For this review, take the finished solid that the model builds, in its own axes (mm). Face numbers are marked on the shaded views. A direction names the side the tool comes from. Give positions to 0.01 mm unless a question says otherwise; leave off trailing zeros. Order: outer loops, then holes, each group sorted by start corner. A loop starts at its lowest first (then second) coordinate and runs counter-clockwise, first axis right, second up.
Item 1: Consider section B-B (y = 2.5). Give the boundary of the cut face in (x, z), plus the area to 3 significant figures.
Item 2: For P1, Ø6, axis at x = 5, y = 3, coming from the +Z side; P2, Ø1.5, axis at y = 3, z = -7.5, coming from the +X side, all flat-tipped, find the tip position at first contact; note any pin that passes through.
Item 3: Consider section A-A (x = 19.05). Give the boundary of the cut face in (y, z), plus the area to 3 significant figures.
Item 4: Consider section C-C (z = -6.5). Give the boundary of the cut face in (x, y), plus the area to 3 significant figures.
Item 5: Consider section D-D (z = -13.5). Give the boundary of the cut face in (x, y) (3 decimals).
Item 6: The part is to be moulded in two halves that separate along Y. For the marked faces 1, 2 and 3, say which applies: released by +Y, released by -Y, zero draft, split by the parting line, or undercut.
Item 7: Machinability: for the marked faces 4 and 5, which of the approach directions +Z, -Z, +X, -X, +Y, -Y give a long, thin tool a straight path to every point of the face, cutting with its end or side? Answer none if there is none.
Item 8: For probe 1 along Z at (x, y) = (3, 10.5); probe 2 along Y at (x, z) = (19.05, -12.55); probe 3 along Z at (x, y) = (12.25, 12.25), list the stretches that pass through material, from the lowest coordinate up.
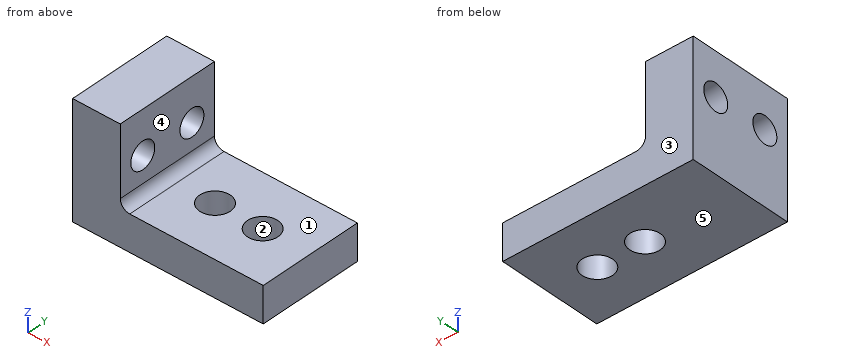
Autodesk Inventor part; units mm, degrees
ref_plane "YZ Plane" through (0, 0, 0) normal (1, 0, 0) x (0, 1, 0)
ref_plane "XZ Plane" through (0, 0, 0) normal (0, 1, 0) x (-1, 0, 0)
ref_plane "XY Plane" through (0, 0, 0) normal (0, 0, 1) x (1, 0, 0)
sketch "Sketch1" plane through (0, 0, 0) normal (1, 0, 0) x (0, 1, 0)
  line L0 (0, 0) -> (13.97, 0)
  line L1 (13.97, 0) -> (13.97, -15.24)
  line L2 (13.97, -15.24) -> (0, -15.24)
  line L3 (0, -15.24) -> (0, 0)
  dimension "d0" = 13.97
  dimension "d1" = 15.24
extrude "Extrusion1" add sketch "Sketch1" along normal blind 6.35
sketch "Sketch2" plane through (6.35, 0, 0) normal (1, 0, 0) x (0, 0, -1)
  line L0 (15.24, 0) -> (15.24, 13.97)
  line L1 (0, 0) -> (15.24, 0)
  line L2 (15.24, 13.97) -> (10.4775, 13.97)
  line L3 (10.4775, 13.97) -> (10.4775, 0)
  line L4 (10.4775, 0) -> (15.24, 0)
  line L5 (15.24, 0) -> (15.24, 13.97)
  dimension "d4" = 4.7625
extrude "Extrusion2" add sketch "Sketch2" along normal blind 19.05
sketch "Sketch3" plane through (6.35, 0, 0) normal (1, 0, 0) x (0, 0, -1)
  line L0 (15.24, 0) -> (0, 0)
  line L1 (0, 0) -> (5.715, 0)
  line L2 (5.715, 0) -> (5.715, 3.3401)
  line L3 (0, 13.97) -> (15.24, 13.97)
  line L4 (5.715, 13.97) -> (5.715, 10.6299)
  line L5 (0, 13.97) -> (0, 0)
  line L6 (15.24, 0) -> (15.24, 13.97)
  dimension "d28" = 9.525
  dimension "d29" = 9.525
  dimension "d30" = 7.2898
  dimension "d31" = 3.3401
  dimension "d32" = 13.97
hole "Hole1" at (6.35, 10.6299, -5.715) at (6.35, 3.3401, -5.715) direction (-1, 0, 0) diameter 3.556 depth 25.4 tip angle 118
fillet "Fillet1" radius 1.27 1 edges at (6.35, 6.985, -10.4775)
sketch "Sketch4" plane through (25.4, 0, -10.4775) normal (0, 0, 1) x (1, 0, 0)
  line L0 (-17.78, 0) -> (0, 0)
  line L1 (0, 0) -> (0, 6.985)
  line L2 (0, 13.97) -> (0, 0)
  line L3 (0, 6.985) -> (-6.35, 6.985)
  line L4 (-19.05, 13.97) -> (-19.05, 0)
  line L5 (-19.05, 6.985) -> (-12.7, 6.985)
  point P0 (-25.4, 0)
  dimension "d19" = 6.35
  dimension "d20" = 6.35
hole "Hole2" at (19.05, 6.985, -10.4775) at (12.7, 6.985, -10.4775) direction (0, 0, -1) diameter 4.064 depth 25.4 tip angle 118
properties part number "GlyphLiftHolder1"
Resolved:
1. outline: (0, -15.24) - (25.4, -15.24) - (25.4, -10.48) - (7.62, -10.48) arc R1.27 cw to (6.35, -9.21) - (6.35, -7.28) - (0, -7.28) - close; (0, -4.15) - (6.35, -4.15) - (6.35, 0) - (0, 0) - close
1. area: 168 mm2
2. P1: stops at z = 0
2. P2: stops at x = 6.35
3. outline: (0, -15.24) - (4.95, -15.24) - (4.95, -10.48) - (0, -10.48) - close; (9.02, -15.24) - (13.97, -15.24) - (13.97, -10.48) - (9.02, -10.48) - close
3. area: 47.2 mm2
4. outline: (0, 0) - (6.35, 0) - (6.35, 1.74) - (0, 1.74) - close; (0, 4.94) - (6.35, 4.94) - (6.35, 9.03) - (0, 9.03) - close; (0, 12.23) - (6.35, 12.23) - (6.35, 13.97) - (0, 13.97) - close
4. area: 48.2 mm2
5. outline: (0, 0) - (25.4, 0) - (25.4, 13.97) - (0, 13.97) - close; hole circle Ø4.064 at (12.7, 6.985); hole circle Ø4.064 at (19.05, 6.985)
6. face 1: zero draft
6. face 2: undercut
6. face 3: released by +Y
7. face 4: +Z, +X, +Y, -Y
7. face 5: -Z, +X, -X, +Y, -Y
8. probe 1: z = -15.24 to -7.49, -3.94 to 0
8. probe 2: y = 0 to 4.95, 9.02 to 13.97
8. probe 3: z = -15.24 to -10.48
